Work out the finished part from the listing and answer in its coordinate system (mm). A direction names the side the tool comes from. Round coordinates to 2 decimals unless told otherwise and drop trailing zeros. Write each loop counter-clockwise with the first axis right and the second up, starting at its lowest first coordinate (ties: lowest second). Pieces come first, ordered by that corner, then holes. Notation, with made-up numbers: M -11.75,32.25 L 26.25,32.25 A14 cw 26.25,38.25 Z; hole C 55.5,85.5 d8. An arc over 180 degrees is marked long. Answer in a Markdown table with one row per item.
```python
from build123d import *

# Parameters (mm, degrees)
SALIENTE_EXTRUIR1_DEPTH = 15
CORTAR_EXTRUIR1_REACH   = 98.556
CROQUIS2_R              = 4.5
CORTAR_EXTRUIR2_REACH   = 98.556
CROQUIS3_R              = 4.5


with BuildPart() as part:
    # Croquis1 → Saliente-Extruir1 (new body)
    with BuildSketch(Plane(origin=(0, 0, 0), x_dir=(1, 0, 0), z_dir=(0, 1, 0))):
        with BuildLine():
            Line((47, 0), (-47, 0))
            Line((-47, 0), (-47, 15))
            Line((-47, 15), (-28, 15))
            Line((-28, 15), (-14.594323866, 71.464925816))
            ThreePointArc((-14.594323866, 71.464925816), (0, 83), (14.594323866, 71.464925816))
            Line((14.594323866, 71.464925816), (28, 15))
            Line((28, 15), (47, 15))
            Line((47, 15), (47, 0))
        make_face()
    extrude(amount=SALIENTE_EXTRUIR1_DEPTH)

    # Croquis2 → Cortar-Extruir1 (cut, up to next)
    with BuildSketch(Plane.XY, mode=Mode.PRIVATE) as cortar_extruir1_sk1:
        with Locations((-38, 7.5)):
            Circle(CROQUIS2_R)
    cortar_extruir1_tool1 = extrude(cortar_extruir1_sk1.sketch, amount=-CORTAR_EXTRUIR1_REACH, mode=Mode.PRIVATE) & part.part
    # Croquis2 → Cortar-Extruir1 (cut, up to next)
    with BuildSketch(Plane.XY, mode=Mode.PRIVATE) as cortar_extruir1_sk2:
        with Locations((38, 7.5)):
            Circle(CROQUIS2_R)
    cortar_extruir1_tool2 = extrude(cortar_extruir1_sk2.sketch, amount=-CORTAR_EXTRUIR1_REACH, mode=Mode.PRIVATE) & part.part
    add(cortar_extruir1_tool1.solids().sort_by_distance((-38, 7.5, 0))[0], mode=Mode.SUBTRACT)
    add(cortar_extruir1_tool2.solids().sort_by_distance((38, 7.5, 0))[0], mode=Mode.SUBTRACT)

    # Croquis3 → Cortar-Extruir2 (cut, up to next)
    with BuildSketch(Plane(origin=(0, 15, 0), x_dir=(1, 0, 0), z_dir=(0, 1, 0)), mode=Mode.PRIVATE) as cortar_extruir2_sk1:
        with Locations(Location((0, 68, 0), (0, 0, 270))):
            Circle(CROQUIS3_R)
    cortar_extruir2_tool1 = extrude(cortar_extruir2_sk1.sketch, amount=-CORTAR_EXTRUIR2_REACH, mode=Mode.PRIVATE) & part.part
    # Croquis3 → Cortar-Extruir2 (cut, up to next)
    with BuildSketch(Plane(origin=(0, 15, 0), x_dir=(1, 0, 0), z_dir=(0, 1, 0)), mode=Mode.PRIVATE) as cortar_extruir2_sk2:
        with Locations(Location((0, 51.9, 0), (0, 0, 270))):
            Circle(CROQUIS3_R)
    cortar_extruir2_tool2 = extrude(cortar_extruir2_sk2.sketch, amount=-CORTAR_EXTRUIR2_REACH, mode=Mode.PRIVATE) & part.part
    add(cortar_extruir2_tool1.solids().sort_by_distance((0, 15, -68))[0], mode=Mode.SUBTRACT)
    add(cortar_extruir2_tool2.solids().sort_by_distance((0, 15, -51.9))[0], mode=Mode.SUBTRACT)


solid = part.part
```
1. Given pin 1 (4 mm diameter, centred on y = 5.5, z = -28.5, fed in from -X); pin 2 (6 mm diameter, centred on y = 13.5, z = -62, fed in from -X); pin 3 (14.5 mm diameter, centred on x = 0, z = -51.9, fed in from -Y); pin 4 (7.5 mm diameter, centred on x = 33, y = 4.5, fed in from -Z), each flat-ended and moving along its own axis, determine where each tip first touches the part or whether it passes through.
Calculated:
| item | result |
|---|---|
| pin 1 | stops at x = -25.27 |
| pin 2 | stops at x = -17.55 |
| pin 3 | stops at y = 0 |
| pin 4 | stops at z = -15 |
2. The part is cut by section B-B (y = 7.5). Determine the outline of the cut face in (x, z), plus the area to 3 significant figures.
Calculated:
| item | result |
|---|---|
| outline | M -47,-15 L -42.5,-15 L -42.5,0 L -47,0 Z; M -33.5,-15 L -28,-15 L -14.59,-71.46 A15 ccw 14.59,-71.46 L 28,-15 L 33.5,-15 L 33.5,0 L -33.5,0 Z; M 42.5,-15 L 47,-15 L 47,0 L 42.5,0 Z; hole C 0,-68 d9; hole C 0,-51.9 d9 |
| area | 3,670 mm² |
3. The part is cut by section A-A (x = 0). Determine the outline of the cut face in (y, z).
Calculated:
| item | result |
|---|---|
| outline | M 0,-83 L 15,-83 L 15,-72.5 L 0,-72.5 Z; M 0,-63.5 L 15,-63.5 L 15,-56.4 L 0,-56.4 Z; M 0,-47.4 L 15,-47.4 L 15,0 L 0,0 Z |
4. The part is cut by section C-C (z = -11). Determine the outline of the cut face in (x, y).
Calculated:
| item | result |
|---|---|
| outline | M -47,0 L 47,0 L 47,15 L -47,15 Z; hole C -38,7.5 d9; hole C 38,7.5 d9 |
5. Consider line 1 along Y through (x, z) = (38, -8.25); line 2 along X through (y, z) = (11, -6); line 3 along Z through (x, y) = (42, 12). Determine where each line is inside the solid, lowest interval first. Write a range as from..to.
Calculated:
| item | result |
|---|---|
| line 1 | y = 0..3, 12..15 |
| line 2 | x = -47..-40.83, -35.17..35.17, 40.83..47 |
| line 3 | z = -15..0 |
6. Determine the mould class of faces 1 (the cylindrical face through (0.198, 7.605, -56.396)), 2 (the cylindrical face through (-33.708, 8.852, -7.395)), 3 (the flat face through (1, 0, -33)) for opening direction Y: released by +Y, released by -Y, zero draft, split by the parting line, or undercut.
Calculated:
| item | result |
|---|---|
| face 1 | zero draft |
| face 2 | undercut |
| face 3 | released by -Y |
7. The part is cut by section D-D (x = 38). Determine the outline of the cut face in (y, z), plus the area to 3 significant figures.
Calculated:
| item | result |
|---|---|
| outline | M 0,-15 L 3,-15 L 3,0 L 0,0 Z; M 12,-15 L 15,-15 L 15,0 L 12,0 Z |
| area | 90.0 mm² |
8. A tool of negligible diameter and unlimited length cuts with its end or side. For faces 4 (the flat face through (1, 15, -33)), 5 (the flat face through (-33, 7, -15)), 6 (the flat face through (33, 7, -15)), from which of +Z, -Z, +X, -X, +Y, -Y can it reach the whole face along a straight path? Write none if from no direction.
Calculated:
| item | result |
|---|---|
| face 4 | +Z, -Z, +X, -X, +Y |
| face 5 | -Z, -X, +Y, -Y |
| face 6 | -Z, +X, +Y, -Y |
